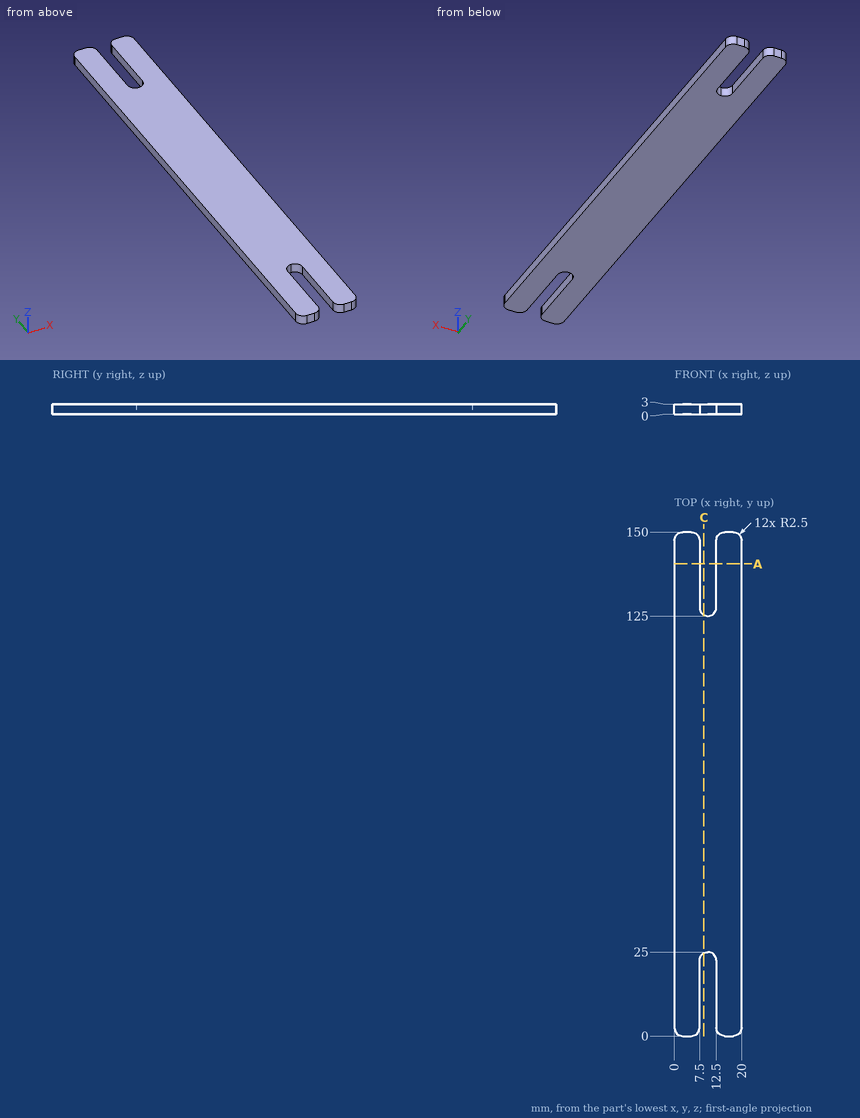
Geometry: see drawing. Coordinates: mm, zero at the bounding-box minimum. Give positions to 0.01 mm unless a question says otherwise; leave off trailing zeros. Order: outer loops, then holes, each group sorted by start corner. A loop starts at its lowest first (then second) coordinate and runs counter-clockwise, first axis right, second up. Notation, with made-up numbers: (-21.75, 66.25) - (-16.75, 66.25) arc R14 cw to (-16.75, 74.25) - close; hole circle Ø6 at (87.5, 37). An arc over 180 degrees is marked (long way). Use a Markdown table: item, result.
(1) Pin query (flat end, axial travel): pin 1 (1.5 mm diameter, centred on x = 11, z = 2, fed in from -Y) (1 decimal). Return the tip coordinate at first contact, or that it passes through.
Computed values:
| item | result |
|---|---|
| pin 1 | stops at y = 24.3 |
(2) Line query: line 1 (X direction, y = 18.5, z = 1.85); line 2 (Y direction, x = 14.75, z = 0.85); line 3 (Y direction, x = 6.25, z = 0.7) (1 decimal). Output: solid intervals per line, ascending. Write a range as from..to.
Computed values:
| item | result |
|---|---|
| line 1 | x = 0..7.5, 12.5..20 |
| line 2 | y = 0.01..149.99 |
| line 3 | y = 0.3..149.7 |
(3) Section query C-C (x = 8.75). Output: boundary loops of the cut face in (y, z) (3 decimals).
Computed values:
| item | result |
|---|---|
| outline | (24.665, 0) - (125.335, 0) - (125.335, 3) - (24.665, 3) - close |
(4) Section query A-A (y = 140.5). Output: boundary loops of the cut face in (x, z), then the cut area to 3 significant figures.
Computed values:
| item | result |
|---|---|
| outline | (0, 0) - (7.5, 0) - (7.5, 3) - (0, 3) - close; (12.5, 0) - (20, 0) - (20, 3) - (12.5, 3) - close |
| area | 45.0 mm2 |
